Could you check a few things on this drawing? It's one solid part, dimensions in mm from its lowest x, y, z. A direction names the side the tool comes from. Give positions to 0.01 mm unless a question says otherwise; leave off trailing zeros. Loops run counter-clockwise (first coordinate to the right, second up) from the corner with the lowest first, then second, coordinate; pieces in that order, holes last.
Q1. Thinking about a two-plate mould opening in Z: for the marked faces 4, 5 and 6, which applies, pulls with the +Z half, pulls with the -Z half, needs draft (parallel to the pull), parting line crosses it, or undercut?
Q2. I need wall thicknesses on probe 1 along Y at (x, z) = (0.7, 5.5); probe 2 along Y at (x, z) = (3.6, 5.5); probe 3 along X at (y, z) = (6.75, 3.5). Which ranges of each line are inside material? Lowest first, please.
Q3. Suppose I cut it at C-C (x = 1.3). List the corners of the cut face in (y, z) for me, and give its area (3 significant figures).
Q4. For the marked faces 1, 2 and 3, which set-ups out of +Z, -Z, +X, -X, +Y, -Y let a thin tool reach every point of the face, with its end or its side?
Q5. Suppose I cut it at A-A (z = 5.5). List the corners of the cut face in (x, y) for me, and give its area (4 significant figures).
Q6. I'm going to push flat-ended pins straight in: P1, Ø1.5, axis at y = 3, z = 3.5, coming from the -X side; P2, Ø1.5, axis at x = 1, z = 2.5, coming from the -Y side. Where does each tip first touch, or does it pass through?
Q7. Suppose I cut it at D-D (y = 8.25). List the corners of the cut face in (x, z) for me, and give its area (3 significant figures).
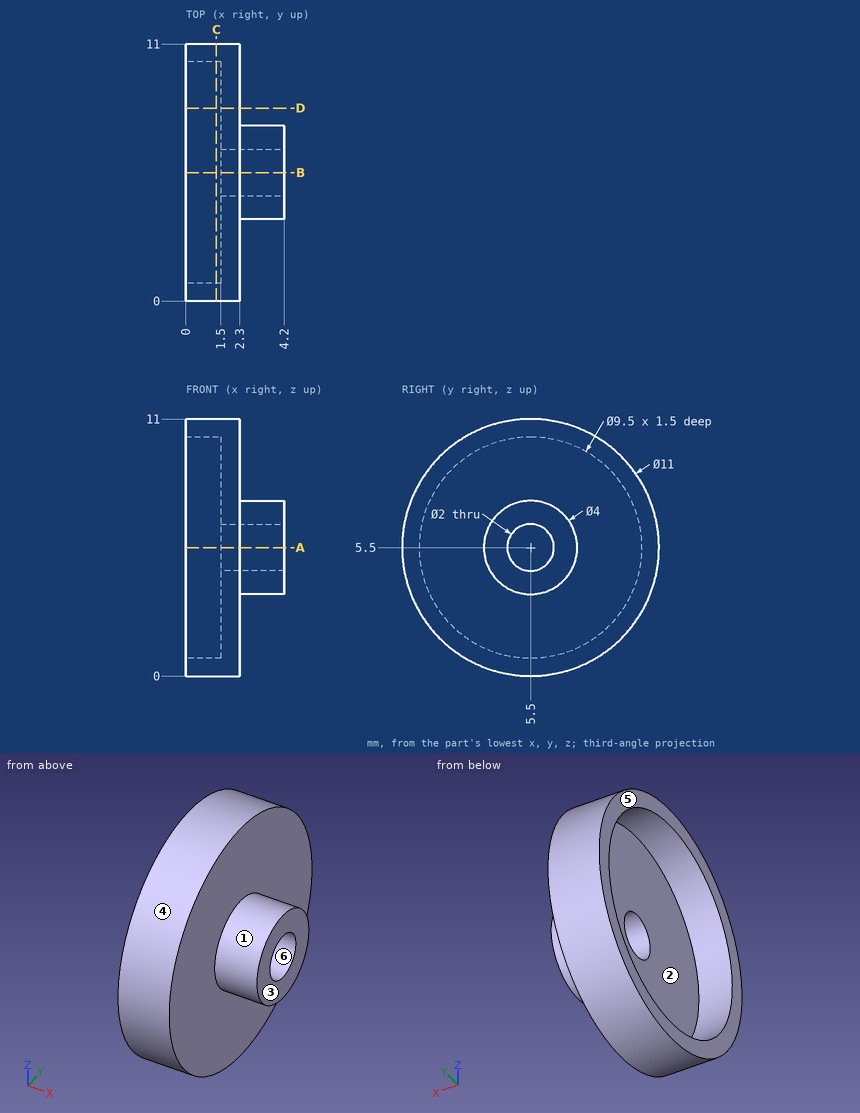
Solutions:
1. face 4: parting line crosses it
1. face 5: needs draft
1. face 6: undercut
2. probe 1: y = 0 to 0.75, 10.25 to 11
2. probe 2: y = 3.5 to 4.5, 6.5 to 7.5
2. probe 3: x = 1.5 to 2.3
3. outline: circle Ø11 at (5.5, 5.5); hole circle Ø9.5 at (5.5, 5.5)
3. area: 24.2 mm2
4. face 1: +X
4. face 2: -X
4. face 3: +Z, -Z, +X, +Y, -Y
5. outline: (0, 0) - (2.3, 0) - (2.3, 3.5) - (4.2, 3.5) - (4.2, 4.5) - (1.5, 4.5) - (1.5, 0.75) - (0, 0.75) - close; (0, 10.25) - (1.5, 10.25) - (1.5, 6.5) - (4.2, 6.5) - (4.2, 7.5) - (2.3, 7.5) - (2.3, 11) - (0, 11) - close
5. area: 13.25 mm2
6. P1: stops at x = 1.5
6. P2: stops at y = 0.48
7. outline: (0, 0.74) - (2.3, 0.74) - (2.3, 10.26) - (0, 10.26) - (0, 9.37) - (1.5, 9.37) - (1.5, 1.63) - (0, 1.63) - close
7. area: 10.3 mm2
